Autodesk Inventor part; units mm, degrees
ref_plane "YZ Plane" through (0, 0, 0) normal (1, 0, 0) x (0, 1, 0)
ref_plane "XZ Plane" through (0, 0, 0) normal (0, 1, 0) x (-1, 0, 0)
ref_plane "XY Plane" through (0, 0, 0) normal (0, 0, 1) x (1, 0, 0)
sketch "Boceto1" plane through (0, 0, 0) normal (0, 1, 0) x (-1, 0, 0)
  circle A0 centre (0, 0) radius 12.7 construction
  circle A1 centre (0, 0) radius 20
  line L0 (0, -12.7) -> (-8.9803, -8.9803)
  line L1 (-8.9803, -8.9803) -> (-12.7, 0)
  line L2 (-12.7, 0) -> (-8.9803, 8.9803)
  line L3 (-8.9803, 8.9803) -> (0, 12.7)
  line L4 (0, 12.7) -> (8.9803, 8.9803)
  line L5 (8.9803, 8.9803) -> (12.7, 0)
  line L6 (12.7, 0) -> (8.9803, -8.9803)
  line L7 (8.9803, -8.9803) -> (0, -12.7)
  point P0 (0, 12.7)
  dimension "d0" = 25.4
  dimension "d1" = 40
extrude "Extrusión1" add sketch "Boceto1" along normal blind 3
properties part number "espaciador"
Model file for the job. Use its own axes, mm. A direction names the side the tool comes from. Give positions to 0.01 mm unless a question says otherwise; leave off trailing zeros. Write each loop counter-clockwise with the first axis right and the second up, starting at its lowest first coordinate (ties: lowest second). Pieces come first, ordered by that corner, then holes. Notation, with made-up numbers: M -3.5,15 L 54.5,15 A24 ccw 54.5,34 Z; hole C 21,-38.5 d11. An arc over 180 degrees is marked long. Use a Markdown table: item, result.
1) Pin check, flat tip, straight feed: pin 1 (1.5 mm diameter, centred on x = -10, y = 1, fed in from -Z). Stop position of the tip, or through.
Responses:
| item | result |
|---|---|
| pin 1 | stops at z = -17.73 |
2) Cut at B-B (x = -1). List the corners of the cut face in (y, z).
Responses:
| item | result |
|---|---|
| outline | M 0,-19.97 L 3,-19.97 L 3,-12.29 L 0,-12.29 Z; M 0,12.29 L 3,12.29 L 3,19.97 L 0,19.97 Z |
3) Cut at C-C (y = 0.75). List the corners of the cut face in (x, z).
Responses:
| item | result |
|---|---|
| outline | C 0,0 d40; hole M -12.7,0 L -8.98,-8.98 L 0,-12.7 L 8.98,-8.98 L 12.7,0 L 8.98,8.98 L 0,12.7 L -8.98,8.98 Z |
4) Drill centre lines: line 1 (Z direction, x = 0, y = 2.15); line 2 (Z direction, x = -1.5, y = 0.5); line 3 (X direction, y = 1.65, z = -4). Where is each one in solid material? Low to high. Write a range as from..to.
Responses:
| item | result |
|---|---|
| line 1 | z = -20..-12.7, 12.7..20 |
| line 2 | z = -19.94..-12.08, 12.08..19.94 |
| line 3 | x = -19.6..-11.04, 11.04..19.6 |
5) Cut at A-A (z = -1). List the corners of the cut face in (x, y), and give its area (3 significant figures).
Responses:
| item | result |
|---|---|
| outline | M -19.97,0 L -12.29,0 L -12.29,3 L -19.97,3 Z; M 12.29,0 L 19.97,0 L 19.97,3 L 12.29,3 Z |
| area | 46.1 mm2 |
6) Pull direction X, two halves, no side cores. Call faces 3 (the flat face through (10.814, 1.479, -4.553)), 4 (the cylindrical face through (4.336, 1.479, 19.524)), 5 (the flat face through (-13, 0, 0)): +X half, -X half, draft (parallel to the pull), parting line (faces both ways), or undercut.
Responses:
| item | result |
|---|---|
| face 3 | undercut |
| face 4 | parting line |
| face 5 | draft |
7) Tool access for faces 1 (the flat face through (-13, 3, 0)), 2 (the flat face through (4.427, 1.479, -10.866)): list every direction of +Z, -Z, +X, -X, +Y, -Y with a clear straight run to the whole face (end or side of a thin tool).
Responses:
| item | result |
|---|---|
| face 1 | +Z, -Z, +X, -X, +Y |
| face 2 | +Y, -Y |
8) Cut at D-D (z = -14.5). List the corners of the cut face in (x, y), and give its area (4 significant figures).
Responses:
| item | result |
|---|---|
| outline | M -13.77,0 L 13.77,0 L 13.77,3 L -13.77,3 Z |
| area | 82.65 mm2 |
